```python
from build123d import *

# Parameters (mm, degrees)
SKETCH003_R     = 8
PAD003_DEPTH    = 40
SKETCH004_R     = 1.5
POCKET_DEPTH    = 13.5
SKETCH005_R     = 7.45
POCKET001_DEPTH = 40.001


with BuildPart() as part:
    # Sketch003 → Pad003 (new body)
    with BuildSketch(Plane.XZ):
        with Locations((0, 15)):
            Circle(SKETCH003_R)
    extrude(amount=-PAD003_DEPTH)

    # Sketch004 (on DatumPlane) → Pocket (cut, symmetric)
    with BuildSketch(Plane.XY.offset(15)):
        with Locations((0, 5)):
            Circle(SKETCH004_R)
    extrude(amount=POCKET_DEPTH, both=True, mode=Mode.SUBTRACT)

    # Sketch005 → Pocket001 (cut, through all)
    with BuildSketch(Plane.XZ):
        with Locations((0, 15)):
            Circle(SKETCH005_R)
    extrude(amount=-POCKET001_DEPTH, mode=Mode.SUBTRACT)


with BuildPart() as part_1:
    # Body003 placement: moved
    add(part.part.moved(Location((0, -11, 0))))


solid = part_1.part
```
Read the model definition and answer for the solid it produces. Units are mm, in the model's axes. Give positions to 0.01 mm unless a question says otherwise; leave off trailing zeros. Write each loop counter-clockwise with the first axis right and the second up, starting at its lowest first coordinate (ties: lowest second). Pieces come first, ordered by that corner, then holes. Notation, with made-up numbers: (-12.5, 81) - (24.5, 81) arc R13 cw to (24.5, 103) - close; hole circle Ø2 at (-17.75, -6). An arc over 180 degrees is marked (long way). Write item = value, one per line. Start each with the question number.
Item 1: Find section A-A (x = 0). Give the vertices of the cut face in (y, z), then the cut area to 3 significant figures.
Item 2: Find section C-C (x = -5). Give the vertices of the cut face in (y, z) (3 decimals), then the cut area to 3 significant figures.
Item 3: Find section B-B (z = 14.5). Give the vertices of the cut face in (x, y).
Item 4: Each of these flat-tipped pins is pushed along its axis until it touches: P1, Ø6, axis at x = -4, y = 22, coming from the -Z side; P2, Ø5, axis at x = 0, y = -6, coming from the +Z side; P3, Ø4, axis at x = -5, z = 14.5, coming from the -Y side; P4, Ø3, axis at y = 20, z = 10, coming from the +X side. Where does it stop, or does it pass through?
Item 5: Find the intervals of material crossed by probe 1 along Y at (x, z) = (0, 22.5); probe 2 along Z at (x, y) = (0, 12); probe 3 along Z at (x, y) = (-4.75, 1), in increasing order. Write a range as [from, to].
Item 6: Find section D-D (y = -2.5). Give the vertices of the cut face in (x, z), then the cut area to 3 significant figures.
Response:
q1.outline = (-11, 7) - (-7.5, 7) - (-7.5, 7.55) - (-11, 7.55) - close; (-11, 22.45) - (-7.5, 22.45) - (-7.5, 23) - (-11, 23) - close; (-4.5, 7) - (29, 7) - (29, 7.55) - (-4.5, 7.55) - close; (-4.5, 22.45) - (29, 22.45) - (29, 23) - (-4.5, 23) - close
q1.area = 40.7 mm²
q2.outline = (-11, 8.755) - (29, 8.755) - (29, 9.477) - (-11, 9.477) - close; (-11, 20.523) - (29, 20.523) - (29, 21.245) - (-11, 21.245) - close
q2.area = 57.8 mm²
q3.outline = (-7.98, -11) - (-7.43, -11) - (-7.43, 29) - (-7.98, 29) - close; (7.43, -11) - (7.98, -11) - (7.98, 29) - (7.43, 29) - close
q4.P1 = 7.06
q4.P2 = 23
q4.P3 = through
q4.P4 = 7.19
q5.probe_1 = [-11, -7.5], [-4.5, 29]
q5.probe_2 = [7, 7.55], [22.45, 23]
q5.probe_3 = [8.56, 9.26], [20.74, 21.44]
q6.outline = circle Ø16 at (0, 15); hole circle Ø14.9 at (0, 15)
q6.area = 26.7 mm²
